Here's how the part is built. I have some questions about the finished solid (model axes, mm). Face numbers are marked on the shaded views. A direction names the side the tool comes from. Round coordinates to 2 decimals unless told otherwise and drop trailing zeros. Order: outer loops, then holes, each group sorted by start corner. A loop starts at its lowest first (then second) coordinate and runs counter-clockwise, first axis right, second up. Notation, with made-up numbers: (43.5, -16.75) -> (56.5, -16.75) arc R15 cw to (56.5, -4.75) -> close; hole circle Ø9 at (32, -23.75). An arc over 180 degrees is marked (long way). Use a Markdown table: item, result. Add a question column.
(1) Thinking about a two-plate mould opening in X: for the marked faces 4, 5 and 6, which applies, pulls with the +X half, pulls with the -X half, needs draft (parallel to the pull), parting line crosses it, or undercut?
(2) I want a section at A-A, the plane y = 0. Please give me the cut outline in (x, z), then the cut area to 3 significant figures.
(3) If I drill on probe 1 along X at (y, z) = (228, 1585); probe 2 along Z at (x, y) = (583.5, -339.5); probe 3 along X at (y, z) = (325, 632), over which ranges is the centre line in solid material (lowest first)?
(4) I'm going to push flat-ended pins straight in: P1, Ø12, axis at y = 223.5, z = 958.5, coming from the -X side; P2, Ø8, axis at x = 4.5, y = 407, coming from the -Z side; P3, Ø5, axis at x = -544.5, z = 314.5, coming from the +Y side. Where does each tip first touch, or does it pass through?
(5) I want a section at B-B, the plane x = -530. Please give me the cut outline in (y, z).
(6) I want a section at D-D, the plane z = 1521.5. Please give me the cut outline in (x, y).
(7) I want a section at C-C, the plane z = 449. Please give me the cut outline in (x, y), then the cut area to 3 significant figures.
(8) On a 3-axis mill with a long thin cutter (end or side, diameter ignored), from which of +Z, -Z, +X, -X, +Y, -Y can I reach the whole of each face in a straight line? I mean the marked faces 1, 2 and 3. Say none if no direction works.
from build123d import *

# Parameters (mm, degrees)
F0_W      = 1502
F0_H      = 750
F1_DEPTH  = 1376
F3_R      = 78.7473915707
F5_W      = 750
F5_H      = 297.2130477428
F6_DEPTH  = 241
F8_DEPTH  = 1261
F9_DEPTH  = 25
F10_W     = 336.0105156898
F10_H     = 266.2700414658
F11_DEPTH = 10


with BuildPart() as f1:
    # F0 (on Top) → F1 (new body)
    with BuildSketch(Plane.XY):
        Rectangle(F0_W, F0_H)
    extrude(amount=F1_DEPTH)

    # F4: sweep along a path in F2
    with BuildLine(Plane.XZ) as f4_path:
        Line((-751, 1078.6715745926), (-851, 1078.6715745926))
        ThreePointArc((-851, 1078.6715745926), (-921.7106781187, 1049.3822527112), (-951, 978.6715745926))
        Line((-951, 978.6715745926), (-951, 308.378726244))
    # F3 (on face) → F4 (sweep)
    with BuildSketch(Plane(origin=(-751, 0, 0), x_dir=(0, -1, 0), z_dir=(-1, 0, 0))):
        with Locations((0, 1089.3139839172)):
            Circle(F3_R)
    sweep(path=f4_path.line)

    # F5 (on face) → F6 (cut)
    with BuildSketch(Plane.YZ.offset(751)):
        with Locations((0, 148.6065238714)):
            Rectangle(F5_W, F5_H)
    extrude(amount=-F6_DEPTH, mode=Mode.SUBTRACT)

    # F7 (on face) → F8 (join, through all)
    with BuildSketch(Plane.YZ.offset(510)):
        Polygon((-374.2722838136, 1668), (-374.2722838136, 1376), (372.3494112492, 1376), (372.3494112492, 1775.292634964), (267.1647369862, 1960), (-168.9238548279, 1960), align=None)
    extrude(amount=-F8_DEPTH)

    # F9 (add): a face of the model
    f9_faces = [f1.faces().sort_by_distance(p)[0] for p in [
        (-22.6360261364, 375, 707.3651464289),
    ]]
    extrude(f9_faces, amount=F9_DEPTH)

    # F10 (on face) → F11 (join)
    with BuildSketch(Plane(origin=(0, 400, 0), x_dir=(-1, 0, 0), z_dir=(0, 1, 0))):
        with Locations((42.0069694519, 1141.3634419441)):
            Rectangle(F10_W, F10_H)
    extrude(amount=F11_DEPTH)


solid = f1.part
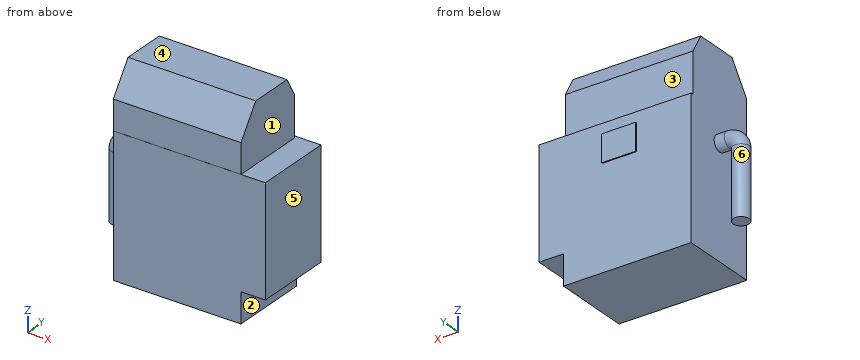
Taken from the geometry:
| question | item | result |
|---|---|---|
| 1 | face 4 | needs draft |
| 1 | face 5 | pulls with the +X half |
| 1 | face 6 | undercut |
| 2 | outline | (-1040.39, 308.38) -> (-882.9, 308.38) -> (-882.9, 978.67) arc R31.9 cw to (-851, 1010.57) -> (-751, 1010.57) -> (-751, 0) -> (510, 0) -> (510, 297.21) -> (751, 297.21) -> (751, 1376) -> (510, 1376) -> (510, 1960) -> (-751, 1960) -> (-751, 1168.06) -> (-851, 1168.06) arc R189.39 ccw to (-1040.39, 978.67) -> close |
| 2 | area | 2,880,000 mm2 |
| 3 | probe 1 | x = -751 to 510 |
| 3 | probe 2 | z = 297.21 to 1376 |
| 3 | probe 3 | x = -751 to 751 |
| 4 | P1 | stops at x = -751 |
| 4 | P2 | stops at z = 1008.23 |
| 4 | P3 | stops at y = 400 |
| 5 | outline | (-375, 0) -> (400, 0) -> (400, 1376) -> (372.35, 1376) -> (372.35, 1775.29) -> (267.16, 1960) -> (-168.92, 1960) -> (-374.27, 1668) -> (-374.27, 1376) -> (-375, 1376) -> close |
| 6 | outline | (-751, -374.27) -> (510, -374.27) -> (510, 372.35) -> (-751, 372.35) -> close |
| 7 | outline | circle Ø157.49 at (-961.64, 0); (-751, -375) -> (751, -375) -> (751, 400) -> (-751, 400) -> close |
| 7 | area | 1,180,000 mm2 |
| 8 | face 1 | +Z, +X, +Y, -Y |
| 8 | face 2 | -Z, +X, +Y, -Y |
| 8 | face 3 | +Z, +X, -X, +Y |
